```python
from build123d import *

# Parameters (mm, degrees)
SKETCH1_R             = 65
SKETCH1_R_2           = 40
SKETCH1_R_3           = 3.05
BOSS_EXTRUDE1_DEPTH   = 15
SKETCH2_R             = 3
CUT_EXTRUDE1_DEPTH    = 94.139680051
CIRPATTERN1_COUNT     = 6
CIRPATTERN2_OUTLINE_R = 3.05
CIRPATTERN2_DEPTH     = 15


# Read off the part's stored shape, not the designer's step: CirPattern2
with BuildPart() as part:
    # Sketch1 → Boss-Extrude1 (new body)
    with BuildSketch(Plane(origin=(0, 0, 0), x_dir=(1, 0, 0), z_dir=(0, 1, 0))):
        with Locations(Location((0, 0, 0), (0, 0, 270))):
            Circle(SKETCH1_R)
        with Locations(Location((0, 0, 0), (0, 0, 270))):
            Circle(SKETCH1_R_2, mode=Mode.SUBTRACT)
        with Locations(Location((12.723046489, -48.354152749, 0), (0, 0, 270))):
            Circle(SKETCH1_R_3, mode=Mode.SUBTRACT)
    extrude(amount=BOSS_EXTRUDE1_DEPTH)

    # Sketch2 → Cut-Extrude1 (cut, through all)
    with BuildSketch(Plane(origin=(0, 0, 0), x_dir=(0, 0, -1), z_dir=(1, 0, 0))):
        with Locations((0, 7.5)):
            Circle(SKETCH2_R)
    cut_extrude1 = extrude(amount=-CUT_EXTRUDE1_DEPTH, mode=Mode.SUBTRACT)

    # CirPattern1: Cut-Extrude1 ×6 about axis
    cirpattern1_axis = Axis((0, 15, 0), (0, 1, 0))
    for i in range(1, CIRPATTERN1_COUNT):
        add(cut_extrude1.rotate(cirpattern1_axis, i * 360 / CIRPATTERN1_COUNT), mode=Mode.SUBTRACT)

    # CirPattern2 outline → CirPattern2 (cut)
    with BuildSketch(Plane(origin=(0, 0, 0), x_dir=(1, 0, 0), z_dir=(0, 1, 0))):
        with Locations((-35.514401414, -35.195557847)):
            Circle(CIRPATTERN2_OUTLINE_R)
        with Locations((-48.237447903, 13.158594901)):
            Circle(CIRPATTERN2_OUTLINE_R)
        with Locations((-12.723046489, 48.354152749)):
            Circle(CIRPATTERN2_OUTLINE_R)
        with Locations((35.514401414, 35.195557847)):
            Circle(CIRPATTERN2_OUTLINE_R)
        with Locations((48.237447903, -13.158594901)):
            Circle(CIRPATTERN2_OUTLINE_R)
    extrude(amount=CIRPATTERN2_DEPTH, mode=Mode.SUBTRACT)


solid = part.part
```
Verification items for the finished model (mm, model axes). Give positions to 0.01 mm unless a question says otherwise; leave off trailing zeros. Order: outer loops, then holes, each group sorted by start corner. A loop starts at its lowest first (then second) coordinate and runs counter-clockwise, first axis right, second up. Notation, with made-up numbers: (71.25, 85) -> (80.25, 85) arc R26 ccw to (80.25, 104) -> close; hole circle Ø3 at (55, 12.25). An arc over 180 degrees is marked (long way). Use a Markdown table: item, result.
1) Section check C-C, the plane y = 7.5. Give the number of separate pieces and of enclosed holes in the cut face, then the cut area to 3 significant figures.
Results:
| item | result |
|---|---|
| separate pieces | 6 |
| enclosed holes | 6 |
| area | 7,170 mm² |
2) Section check B-B, the plane z = 0. Record the boundary of the cut face in (x, y).
Results:
| item | result |
|---|---|
| outline | (-65, 0) -> (-40, 0) -> (-40, 4.5) -> (-65, 4.5) -> close; (-65, 10.5) -> (-40, 10.5) -> (-40, 15) -> (-65, 15) -> close; (40, 0) -> (65, 0) -> (65, 4.5) -> (40, 4.5) -> close; (40, 10.5) -> (65, 10.5) -> (65, 15) -> (40, 15) -> close |
3) Mould release check, pull along Y, two halves, no side actions. Record for faces 1 (the cylindrical face through (13.639, 7.395, 51.263)), 2 (the cylindrical face through (28.73, 7.63, 43.77)), 3 (the flat face through (30, 15, 28)): pulls with the +Y half, pulls with the -Y half, needs draft (parallel to the pull), parting line crosses it, or undercut.
Results:
| item | result |
|---|---|
| face 1 | needs draft |
| face 2 | undercut |
| face 3 | pulls with the +Y half |
4) Depth check by flat-ended pin: pin 1 Ø5 at (x, z) = (48.24, 13.16) entering from -Y; pin 2 Ø6 at (x, y) = (-6, 7.5) entering from -Z; pin 3 Ø1 at (x, y) = (13, 4.5) entering from -Z; pin 4 Ø4 at (x, y) = (-14, 3) entering from +Z. Enter the tip coordinate at first touch or a pass-through.
Results:
| item | result |
|---|---|
| pin 1 | through |
| pin 2 | z = -64.93 |
| pin 3 | z = -63.79 |
| pin 4 | z = 63.88 |
5) Section check A-A, the plane x = 0. Record the boundary of the cut face in (y, z), then the cut area to 3 significant figures.
Results:
| item | result |
|---|---|
| outline | (0, -65) -> (15, -65) -> (15, -40) -> (0, -40) -> close; (0, 40) -> (15, 40) -> (15, 65) -> (0, 65) -> close |
| area | 750 mm² |
6) Material ranges on probe 1 along X at (y, z) = (7, -44); probe 2 along X at (y, z) = (7, -46.5); probe 3 along Z at (x, y) = (37, 7.5), recorded low to high.
Results:
| item | result |
|---|---|
| probe 1 | -47.84 to -28.82, -21.99 to 21.99, 28.82 to 47.84 |
| probe 2 | -45.42 to -30.26, -23.43 to -15.14, -10.3 to 23.43, 30.26 to 45.42 |
| probe 3 | -53.44 to -37.86, -32.53 to -15.2, 15.2 to 53.44 |
7) Section check D-D, the plane z = 23. Record the boundary of the cut face in (x, y), then the cut area to 3 significant figures.
Results:
| item | result |
|---|---|
| outline | (-60.79, 0) -> (-32.73, 0) -> (-32.73, 15) -> (-60.79, 15) -> close; (32.73, 0) -> (60.79, 0) -> (60.79, 15) -> (32.73, 15) -> close |
| area | 842 mm² |
